Here's how the part is built. I have some questions about the finished solid (model axes, mm). A direction names the side the tool comes from. Coordinates: 2 decimals unless noted, no trailing zeros. Order: outer loops, then holes, each group sorted by start corner. A loop starts at its lowest first (then second) coordinate and runs counter-clockwise, first axis right, second up. Notation, with made-up numbers: (24.5, -33.75) - (36.5, -33.75) arc R8 ccw to (36.5, -20.75) - close; hole circle Ø7 at (-10, -4). An arc over 180 degrees is marked (long way). Use CSV: the item, a comma, the result in double quotes. Start each with the question number.
from build123d import *

# Parameters (mm, degrees)
F0_W      = 420
F0_H      = 420
F1_DEPTH  = 105
F2_T      = -6
F3_W      = 6
F3_H      = 408
F4_DEPTH  = 18
F5_W      = 6
F5_H      = 408
F6_DEPTH  = 18
F7_W      = 6
F7_H      = 18
F8_DEPTH  = 372
F9_W      = 6
F9_H      = 18
F10_DEPTH = 372
F11_W     = 408
F11_H     = 408
F11_W_2   = 400
F11_H_2   = 400
F12_DEPTH = 10
F13_W     = 400
F13_H     = 200
F14_DEPTH = 10


with BuildPart() as f1:
    # F0 (on Front) → F1 (new body, symmetric)
    with BuildSketch(Plane.XZ):
        Rectangle(F0_W, F0_H)
    extrude(amount=F1_DEPTH, both=True)

    # F2
    f2_openings = [f1.faces().sort_by_distance(p)[0] for p in [
        (0, -105, 0),
    ]]
    offset(amount=F2_T, openings=f2_openings)

    # F3 (on face) → F4 (join)
    with BuildSketch(Plane.YZ.offset(-204)):
        with Locations((-92, 0)):
            Rectangle(F3_W, F3_H)
    extrude(amount=F4_DEPTH)

    # F5 (on face) → F6 (join)
    with BuildSketch(Plane(origin=(204, 0, 0), x_dir=(0, -1, 0), z_dir=(-1, 0, 0))):
        with Locations((92, 0)):
            Rectangle(F5_W, F5_H)
    extrude(amount=F6_DEPTH)

    # F7 (on face) → F8 (join, through all)
    with BuildSketch(Plane.YZ.offset(-186)):
        with Locations((-92, 195)):
            Rectangle(F7_W, F7_H)
    extrude(amount=F8_DEPTH)

    # F9 (on face) → F10 (join, through all)
    with BuildSketch(Plane.YZ.offset(-186)):
        with Locations((-92, -195)):
            Rectangle(F9_W, F9_H)
    extrude(amount=F10_DEPTH)

    # F11 (on face) → F12 (join)
    with BuildSketch(Plane.XZ.offset(95)):
        Rectangle(F11_W, F11_H)
        Rectangle(F11_W_2, F11_H_2, mode=Mode.SUBTRACT)
    extrude(amount=F12_DEPTH)

    # F13 (on face) → F14 (join)
    with BuildSketch(Plane.XZ.offset(95)):
        with Locations((0, -100)):
            Rectangle(F13_W, F13_H)
    extrude(amount=F14_DEPTH)


solid = f1.part
Item 1: Suppose I cut it at D-D on z = 119. Write out the boundary of the cut face in (x, y), then the cut area to 3 significant figures.
Item 2: For faces 5 (the flat face through (195, -89, -16)), 6 (the flat face through (200, -100, 99)), 7 (the flat face through (-3, -1, 210)), which set-ups out of +Z, -Z, +X, -X, +Y, -Y let a thin tool reach every point of the face, with its end or its side?
Item 3: For pin 1 Ø8 at (x, z) = (-39, 108.5) entering from -Y, with a flat end and sliding along its axis, tell me the tip position at first contact or that it passes through.
Item 4: Suppose I cut it at B-B on y = 32. Write out the boundary of the cut face in (x, z).
Item 5: Suppose I cut it at A-A on z = -130. Write out the boundary of the cut face in (x, y), then the cut area to 3 significant figures.
Item 6: We'd pull the mould along Y, two halves only. Please class faces 1 (the flat face through (-204, 4, -3)), 2 (the flat face through (-3, 105, 3)), 3 (the flat face through (-3, -100, 0)), 4 (the flat face through (-1, -95, 188)): released by +Y, released by -Y, zero draft, split by the parting line, or undercut.
Item 7: Please list where these lines run through material, in increasing order: line 1 along X through (y, z) = (69, 41); line 2 along Y through (x, z) = (-153, -112); line 3 along Y through (x, z) = (-189.5, 81.5). Write a range as from..to.
Item 8: Suppose I cut it at C-C on x = -140.5. Write out the boundary of the cut face in (y, z), then the cut area to 3 significant figures.
Here are the results:
1,outline,"(-210, -105) - (-200, -105) - (-200, -95) - (-186, -95) - (-186, -89) - (-204, -89) - (-204, 99) - (204, 99) - (204, -89) - (186, -89) - (186, -95) - (200, -95) - (200, -105) - (210, -105) - (210, 105) - (-210, 105) - close"
1,area,"5,260 mm^2"
2,face 5,"none"
2,face 6,"-Y"
2,face 7,"+Z, +X, -X, +Y, -Y"
3,pin 1,"y = 99"
4,outline,"(-210, -210) - (210, -210) - (210, 210) - (-210, 210) - close; hole (-204, -204) - (204, -204) - (204, 204) - (-204, 204) - close"
5,outline,"(-210, -105) - (210, -105) - (210, 105) - (-210, 105) - close; hole (-204, -89) - (-186, -89) - (-186, -95) - (186, -95) - (186, -89) - (204, -89) - (204, 99) - (-204, 99) - close"
5,area,"9,260 mm^2"
6,face 1,"undercut"
6,face 2,"released by +Y"
6,face 3,"zero draft"
6,face 4,"released by -Y"
7,line 1,"-210..-204, 204..210"
7,line 2,"-105..-95, 99..105"
7,line 3,"-95..-89, 99..105"
8,outline,"(-105, -210) - (105, -210) - (105, 210) - (-105, 210) - (-105, 200) - (-95, 200) - (-95, 186) - (-89, 186) - (-89, 204) - (99, 204) - (99, -204) - (-89, -204) - (-89, -186) - (-95, -186) - (-95, 0) - (-105, 0) - close"
8,area,"7,260 mm^2"
